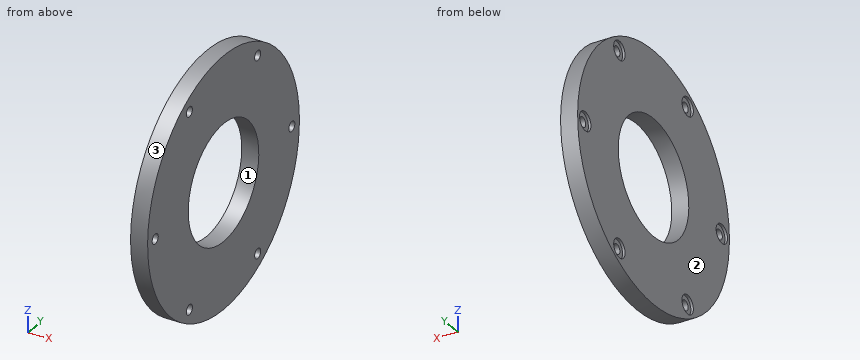
```python
from build123d import *

# Parameters (mm, degrees)
SKETCH1_R           = 100
SKETCH1_R_2         = 46.5
BOSS_EXTRUDE1_DEPTH = 13.6
HOLE1_D             = 8
HOLE1_DEPTH         = 15
HOLE1_CBORE_D       = 15
HOLE1_CBORE_DEPTH   = 2
HOLE1_TIP           = 2.403442476


with BuildPart() as part:
    # Sketch1 → Boss-Extrude1 (new body)
    with BuildSketch(Plane(origin=(0, 0, 0), x_dir=(0, 0, -1), z_dir=(1, 0, 0))):
        Circle(SKETCH1_R)
        Circle(SKETCH1_R_2, mode=Mode.SUBTRACT)
    extrude(amount=BOSS_EXTRUDE1_DEPTH)

    # Hole1
    with Locations(Plane.ZY):
        with Locations((-77.942286341, 45), (0, 90), (77.942286341, 45), (77.942286341, -45), (0, -90), (-77.942286341, -45)):
            CounterBoreHole(HOLE1_D / 2, HOLE1_CBORE_D / 2, HOLE1_CBORE_DEPTH, depth=HOLE1_DEPTH)
            with Locations((0, 0, -(HOLE1_DEPTH + HOLE1_TIP / 2))):  # 118° drill point
                Cone(0, HOLE1_D / 2, HOLE1_TIP, mode=Mode.SUBTRACT)


solid = part.part
```
Geometry check sheet. Reference: the model listing, model coordinates, mm. Face numbers are marked on the shaded views. Give positions to 0.01 mm unless a question says otherwise; leave off trailing zeros. Order: outer loops, then holes, each group sorted by start corner. A loop starts at its lowest first (then second) coordinate and runs counter-clockwise, first axis right, second up.
1. Thickness scan on L1, parallel to Y at x = 5, z = 0; L2, parallel to Y at x = 1.6, z = 0; L3, parallel to Y at x = 10.25, z = 80. Record the ranges inside material, lowest first.
2. Section check D-D, the plane z = 25.5. Enter the section's corners in (x, y), and give its area (3 significant figures).
3. Section check A-A, the plane z = 0. Enter the section's corners in (x, y), and give its area (3 significant figures).
4. Section check B-B, the plane y = 0. Enter the section's corners in (x, z), and give its area (3 significant figures).
5. Release check for a two-part mould opening along Z. For the marked faces 1, 2 and 3 record: pulls with the +Z half, pulls with the -Z half, needs draft (parallel to the pull), parting line crosses it, or undercut.
6. Gauge pin test, flat ends, axial feed: pin 1 Ø4.5 at (y, z) = (-90, -3.5) entering from -X; pin 2 Ø2 at (x, y) = (5.5, 36) entering from +Z (3 decimals); pin 3 Ø7 at (y, z) = (-90, 0) entering from -X; pin 4 Ø4 at (y, z) = (7, -66.5) entering from -X. Record the tip position at first contact, or that the pin passes through.
7. Section check C-C, the plane x = 8.25. Enter the section's corners in (y, z), and give its area (3 significant figures).
Values follow:
1. L1: y = -100 to -94, -86 to -46.5, 46.5 to 86, 94 to 100
1. L2: y = -100 to -97.5, -82.5 to -46.5, 46.5 to 82.5, 97.5 to 100
1. L3: y = -60 to -48.43, -41.57 to 41.57, 48.43 to 60
2. outline: (0, -96.69) - (13.6, -96.69) - (13.6, -38.88) - (0, -38.88) - close; (0, 38.88) - (13.6, 38.88) - (13.6, 96.69) - (0, 96.69) - close
2. area: 1,570 mm2
3. outline: (0, -100) - (13.6, -100) - (13.6, -94) - (2, -94) - (2, -97.5) - (0, -97.5) - close; (0, -82.5) - (2, -82.5) - (2, -86) - (13.6, -86) - (13.6, -46.5) - (0, -46.5) - close; (0, 46.5) - (13.6, 46.5) - (13.6, 86) - (2, 86) - (2, 82.5) - (0, 82.5) - close; (0, 97.5) - (2, 97.5) - (2, 94) - (13.6, 94) - (13.6, 100) - (0, 100) - close
3. area: 1,210 mm2
4. outline: (0, -100) - (13.6, -100) - (13.6, -46.5) - (0, -46.5) - close; (0, 46.5) - (13.6, 46.5) - (13.6, 100) - (0, 100) - close
4. area: 1,460 mm2
5. face 1: undercut
5. face 2: needs draft
5. face 3: parting line crosses it
6. pin 1: stops at x = 2
6. pin 2: stops at z = 93.675
6. pin 3: passes through
6. pin 4: stops at x = 0
7. outline: circle Ø200 at (0, 0); hole circle Ø8 at (-90, 0); hole circle Ø8 at (-45, -77.94); hole circle Ø8 at (-45, 77.94); hole circle Ø93 at (0, 0); hole circle Ø8 at (45, -77.94); hole circle Ø8 at (45, 77.94); hole circle Ø8 at (90, 0)
7. area: 24,300 mm2
